Autodesk Inventor part; units mm, degrees
ref_plane "YZ Plane" through (0, 0, 0) normal (1, 0, 0) x (0, 1, 0)
ref_plane "XZ Plane" through (0, 0, 0) normal (0, 1, 0) x (-1, 0, 0)
ref_plane "XY Plane" through (0, 0, 0) normal (0, 0, 1) x (1, 0, 0)
sketch "Esquisse4" plane through (0, 0, 0) normal (0, 1, 0) x (-1, 0, 0)
  line L0 (-8, 163) -> (8, 163)
  line L1 (8, 163) -> (8, -163)
  line L2 (8, -163) -> (-8, -163)
  line L3 (-8, -163) -> (-8, 163)
  line L4 (-8, 163) -> (8, -163) construction
  line L5 (8, 163) -> (-8, -163) construction
  point P0 (0, 0)
  dimension "d26" = 16
  dimension "d27" = 326
extrude "Plaque3" add sketch "Esquisse4" along normal blind 1
sketch "Esquisse5" plane through (7, 1, 163) normal (1, 0, 0) x (0, 1, 0)
  line L0 (0, -326) -> (0, 0)
  line L1 (0, 0) -> (-10, 0)
  line L2 (-10, 0) -> (-10, -326)
  line L3 (-10, -326) -> (0, -326)
edge flange "Bord tombé2" height 10 angle 90 thickness 1 bend radius 1 thickness toward (1, 0, 0) relief tear relief width 1 relief depth 0.5 corner gap 1 corner form 0 edges at (8, 0, 0) (-8, 0, 0) wall of the first edge with corners at (7, 1, -163) (7, 1, 163) (7, -9, 163) (7, -9, -163)
bend "Pli2"
corner "Coin2"
sketch "Esquisse6" plane through (0, 1, 0) normal (0, 1, 0) x (1, 0, 0)
  line L0 (-6, 163) -> (6, 163)
  point P0 (0, 0)
  point P1 (0, 158)
  point P2 (0, 163)
  dimension "d39" = 5
hole "Perçage2" at (0, 1, -158) direction (0, -1, 0) diameter 4.5 depth 1
sketch "Esquisse7" plane through (0, 1, 0) normal (0, 1, 0) x (1, 0, 0)
  line L0 (-6, 163) -> (6, 163)
  point P0 (0, 0)
  point P1 (0, -57)
  point P2 (0, -157)
  dimension "d50" = 220
  dimension "d51" = 100
hole "Perçage3" at (0, 1, 57) at (0, 1, 157) direction (0, -1, 0) diameter 4.5 depth 1
sketch "Esquisse8" plane through (8, -9, 163) normal (1, 0, 0) x (0, 0, -1)
  line L0 (326, 8) -> (0, 8)
  line L1 (0, 0) -> (0, 8)
  line L2 (326, 0) -> (0, 0)
  line L3 (326, 8) -> (326, 0)
  line L4 (326, 8) -> (326, 0)
  point P0 (163, 9)
  point P1 (326, 4)
  point P2 (326, 4)
  point P3 (316, 4)
  point P4 (326, 4)
  point P5 (306, 4)
  dimension "d60" = 10
  dimension "d71" = 10
hole "Perçage4" at (8, -5, -153) at (8, -5, -143) direction (-1, 0, 0) diameter 3.4 depth 16
sketch "Esquisse9" plane through (8, -9, 163) normal (1, 0, 0) x (0, 0, -1)
  line L0 (326, 8) -> (326, 0)
  point P0 (163, 9)
  point P1 (226, 4)
  point P2 (326, 4)
  dimension "d72" = 100
hole "Perçage5" at (8, -5, -63) direction (-1, 0, 0) diameter 3.4 depth 16
pattern_linear "Réseau rectangulaire2" count 7 spacing 18 along (0, 0, 1) of "Perçage5"
equation "\"d45\" = Epaisseur"
equation "\"d57\" = Epaisseur"
equation "\"d66\" = Epaisseur"
equation "\"d78\" = Epaisseur"
equation "\"d28\" = Epaisseur"
equation "\"d29\" = LargeurGrugeage"
equation "\"d30\" = ProfondeurGrugeage"
equation "\"d31\" = RestesMinimum"
equation "\"d32\" = Rayondetransition"
equation "\"d35\" = RayonPli"
equation "\"d36\" = TailleGrugeage"
equation "\"d37\" = TailleJeu"
equation "\"d38\" = TailleRayonJacobi"
equation "\"RayonPli\" = Epaisseur"
equation "\"LargeurGrugeage\" = Epaisseur"
equation "\"ProfondeurGrugeage\" = 0.5 * Epaisseur"
equation "\"TailleGrugeage\" = 4 * Epaisseur"
equation "\"RestesMinimum\" = 2 * Epaisseur"
equation "\"Rayondetransition\" = RayonPli"
equation "\"TailleRayonJacobi\" = RayonPli"
equation "\"TailleJeu\" = Epaisseur"
properties part number "support_principal"
Verification items for the finished model (mm, model axes). A direction names the side the tool comes from. Give positions to 0.01 mm unless a question says otherwise; leave off trailing zeros. Loops run counter-clockwise (first coordinate to the right, second up) from the corner with the lowest first, then second, coordinate; pieces in that order, holes last. Notation, with made-up numbers: (76, -12.75) - (130, -12.75) arc R25 cw to (130, 8.25) - close; hole circle Ø9 at (57, 13.25). An arc over 180 degrees is marked (long way). Write each question's results on one line, items separated by ' | '.
1) Depth check by flat-ended pin: P1, Ø2, axis at y = -5, z = 27, coming from the -X side; P2, Ø5, axis at x = 0, z = 57, coming from the -Y side. Enter the tip coordinate at first touch or a pass-through.
Solution:
P1: through | P2: y = 0
2) Sectioned sample at A-A on z = -72.5. Record the boundary of the cut face in (x, y).
Solution:
outline: (-8, -9) - (-7, -9) - (-7, -1) arc R1 cw to (-6, 0) - (6, 0) arc R1 cw to (7, -1) - (7, -9) - (8, -9) - (8, -1) arc R2 ccw to (6, 1) - (-6, 1) arc R2 ccw to (-8, -1) - close
3) Mould release check, pull along X, two halves, no side actions. Record for faces 1 (the flat face through (-7, -5, -2)), 2 (the flat face through (0, 1, 2)), 3 (the flat face through (-8, -5, -2)), 4 (the flat face through (7, -5, 2)): pulls with the +X half, pulls with the -X half, needs draft (parallel to the pull), parting line crosses it, or undercut.
Solution:
face 1: undercut | face 2: needs draft | face 3: pulls with the -X half | face 4: undercut
4) Material ranges on L1, parallel to Z at x = 0, y = 0.8; L2, parallel to X at y = -2, z = 69; L3, parallel to Y at x = -2, z = 120.5, recorded low to high. Write a range as from..to.
Solution:
L1: -163..-160.25, -155.75..54.75, 59.25..154.75, 159.25..163 | L2: -8..-7, 7..8 | L3: 0..1
5) Tool access check on faces 5 (the flat face through (0, 0, 2)), 6 (the flat face through (0.6, 0.4, -163)). Record the directions out of +Z, -Z, +X, -X, +Y, -Y that give a thin tool (end or side, any length) a straight path to the whole face; none if there is none.
Solution:
face 5: +Z, -Z, -Y | face 6: -Z, +X, -X, +Y, -Y
